Build history of the part. All positions in model axes, mm. A direction names the side the tool comes from. Coordinates: 2 decimals unless noted, no trailing zeros. Write each loop counter-clockwise with the first axis right and the second up, starting at its lowest first coordinate (ties: lowest second). Pieces come first, ordered by that corner, then holes.
from build123d import *
from build123d.topology import SkipClean

# Parameters (mm, degrees)
SKETCH_1_W               = 5
SKETCH_1_H               = 10
EXTRUDE_1_DEPTH          = 5.5
SKETCH_3_W               = 5
SKETCH_3_H               = 46.066203836
SKETCH_3_H_2             = 44
EXTRUDE_2_DEPTH          = 44
CUT_EXTRUDE_1_DEPTH      = 316.357337
CUT_EXTRUDE_1_DEPTH_BACK = 316.357337
SKETCH_4_R               = 8.2
SKETCH_4_R_2             = 1.7
SKETCH_5_R               = 15.5
CUT_EXTRUDE_3_DEPTH      = 1.9
CUT_EXTRUDE_START        = -1.9
SKETCH_6_R               = 15.5
CUT_EXTRUDE_4_DEPTH      = 1.9
CUT_EXTRUDE_5_DEPTH      = 316.357337
CUT_EXTRUDE_5_DEPTH_BACK = 316.357337
SKETCH_7_R               = 8.2
SKETCH_7_R_2             = 1.7
SKETCH_8_R               = 15.5
CUT_EXTRUDE_6_DEPTH      = 1.9
SKETCH_9_R               = 15.5
CUT_EXTRUDE_7_DEPTH      = 1.9
SKETCH_10_W              = 10
SKETCH_10_H              = 34
EXTRUDE_3_DEPTH          = 5
SKETCH_11_W              = 5
SKETCH_11_H              = 41.066203836
SKETCH_11_H_2            = 5
SKETCH_11_H_3            = 44
EXTRUDE_4_DEPTH          = 44
CUT_EXTRUDE_8_DEPTH      = 315.095304008
CUT_EXTRUDE_8_DEPTH_BACK = 315.095304008
SKETCH_12_R              = 1.7
SKETCH_12_R_2            = 8.2
SKETCH_17_W              = 210
SKETCH_17_H              = 49.493882771
EXTRUDE_5_DEPTH          = 7.424621
EXTRUDE_6_DEPTH          = 10
EXTRUDE_8_DEPTH          = 10
SKETCH_20_W              = 40
SKETCH_20_H              = 48.239190952
CUT_EXTRUDE_9_DEPTH      = 10
EXTRUDE_11_DEPTH         = 5
EXTRUDE_13_DEPTH         = 210
FILLET_1_R               = 10
EXTRUDE_14_DEPTH         = 5
SKETCH_26_W              = 25
SKETCH_26_H              = 90
EXTRUDE_15_DEPTH         = 5.5
FILLET_2_R               = 10
CHAMFER_1_SIZE           = 4
CHAMFER_2_SIZE           = 3
FILLET_3_R               = 3


with BuildPart() as part:
    # 草图1 → 凸台-拉伸1 (new body)
    with BuildSketch(Plane(origin=(0, 0, 0), x_dir=(1, 0, 0), z_dir=(0, 1, 0))):
        Polygon((85, -44), (5, -44), (5, -186), (85, -186), (85, -220), (125, -220), (125, -186), (205, -186), (205, -44), (125, -44), (125, -10), (85, -10), align=None)
        Polygon((3, 0), (0, 0), (0, -10), (5, -10), (5, 0), align=None)
        Polygon((5, -10), (0, -10), (0, -220), (5, -220), (5, -186), (5, -44), align=None)
        Polygon((205, 0), (5, 0), (5, -10), (85, -10), (125, -10), (205, -10), align=None)
        Polygon((210, -10), (205, -10), (205, -44), (205, -186), (205, -220), (210, -220), align=None)
        with Locations((207.5, -5)):
            Rectangle(SKETCH_1_W, SKETCH_1_H)
        Polygon((85, -220), (5, -220), (5, -230), (205, -230), (205, -220), (125, -220), align=None)
        with Locations((2.5, -225)):
            Rectangle(SKETCH_1_W, SKETCH_1_H)
        with Locations((207.5, -225)):
            Rectangle(SKETCH_1_W, SKETCH_1_H)
    extrude(amount=EXTRUDE_1_DEPTH)

    # 草图3 → 凸台-拉伸2 (add)
    with BuildSketch(Plane(origin=(0, 5.5, 0), x_dir=(1, 0, 0), z_dir=(0, 1, 0))):
        with Locations((2.5, -28.033101918)):
            Rectangle(SKETCH_3_W, SKETCH_3_H)
        with Locations((2.5, -203)):
            Rectangle(SKETCH_3_W, SKETCH_3_H_2)
        with Locations((207.5, -203)):
            Rectangle(SKETCH_3_W, SKETCH_3_H_2)
        with Locations((207.5, -28.033101918)):
            Rectangle(SKETCH_3_W, SKETCH_3_H)
    extrude(amount=EXTRUDE_2_DEPTH)

    # 草图4 → 切除-拉伸1 (cut, two sides: drawn at the far end of the back side and taken through both)
    with BuildSketch(Plane.ZY.offset(-CUT_EXTRUDE_1_DEPTH_BACK)):
        with Locations((28.033101918, 27.5)):
            Circle(SKETCH_4_R)
        with Locations((28.033101918, 15.6)):
            Circle(SKETCH_4_R_2)
        with Locations((17.727399613, 33.45)):
            Circle(SKETCH_4_R_2)
        with Locations((38.338804223, 33.45)):
            Circle(SKETCH_4_R_2)
    extrude(amount=CUT_EXTRUDE_1_DEPTH + CUT_EXTRUDE_1_DEPTH_BACK, mode=Mode.SUBTRACT)

    # 草图5 → 切除-拉伸3 (cut)
    with BuildSketch(Plane.ZY):
        with Locations((28.033101918, 27.5)):
            Circle(SKETCH_5_R)
    extrude(amount=-CUT_EXTRUDE_3_DEPTH, mode=Mode.SUBTRACT)

    # 草图6 → 切除-拉伸4 (cut)
    with BuildSketch(Plane(origin=(210, 0, 0), x_dir=(0, 0, -1), z_dir=(1, 0, 0)).offset(CUT_EXTRUDE_START)):
        with Locations(Location((-28.033101918, 27.5, 0), (0, 0, 180))):
            Circle(SKETCH_6_R)
    extrude(amount=CUT_EXTRUDE_4_DEPTH, mode=Mode.SUBTRACT)

    # 草图7 → 切除-拉伸5 (cut, two sides: drawn at the far end of the back side and taken through both)
    with BuildSketch(Plane.ZY.offset(-CUT_EXTRUDE_5_DEPTH_BACK)):
        with Locations((203, 27.5)):
            Circle(SKETCH_7_R)
        with Locations((203, 15.6)):
            Circle(SKETCH_7_R_2)
        with Locations((192.694297695, 33.45)):
            Circle(SKETCH_7_R_2)
        with Locations((213.305702305, 33.45)):
            Circle(SKETCH_7_R_2)
    extrude(amount=CUT_EXTRUDE_5_DEPTH + CUT_EXTRUDE_5_DEPTH_BACK, mode=Mode.SUBTRACT)

    # 草图8 → 切除-拉伸6 (cut)
    with BuildSketch(Plane.ZY):
        with Locations((203, 27.5)):
            Circle(SKETCH_8_R)
    extrude(amount=-CUT_EXTRUDE_6_DEPTH, mode=Mode.SUBTRACT)

    # 草图9 → 切除-拉伸7 (cut)
    with BuildSketch(Plane(origin=(210, 0, 0), x_dir=(0, 0, -1), z_dir=(1, 0, 0)).offset(CUT_EXTRUDE_START)):
        with Locations(Location((-203, 27.5, 0), (0, 0, 180))):
            Circle(SKETCH_9_R)
    extrude(amount=CUT_EXTRUDE_7_DEPTH, mode=Mode.SUBTRACT)

    # 草图10 → 凸台-拉伸3 (add)
    with BuildSketch(Plane(origin=(0, 5.5, 0), x_dir=(1, 0, 0), z_dir=(0, 1, 0))):
        with Locations((200, -27)):
            Rectangle(SKETCH_10_W, SKETCH_10_H)
        with Locations((10, -27)):
            Rectangle(SKETCH_10_W, SKETCH_10_H)
        with Locations((10, -203)):
            Rectangle(SKETCH_10_W, SKETCH_10_H)
        with Locations((200, -203)):
            Rectangle(SKETCH_10_W, SKETCH_10_H)
    extrude(amount=-EXTRUDE_3_DEPTH)

    # 草图11 → 凸台-拉伸4 (add)
    with BuildSketch(Plane(origin=(0, 5.5, 0), x_dir=(1, 0, 0), z_dir=(0, 1, 0))):
        with Locations((7.5, -30.533101918)):
            Rectangle(SKETCH_11_W, SKETCH_11_H)
        with Locations((7.5, -7.5)):
            Rectangle(SKETCH_11_W, SKETCH_11_H_2)
        with Locations((202.5, -7.5)):
            Rectangle(SKETCH_11_W, SKETCH_11_H_2)
        with Locations((202.5, -30.533101918)):
            Rectangle(SKETCH_11_W, SKETCH_11_H)
        with Locations((7.5, -203)):
            Rectangle(SKETCH_11_W, SKETCH_11_H_3)
        with Locations((202.5, -203)):
            Rectangle(SKETCH_11_W, SKETCH_11_H_3)
    extrude(amount=EXTRUDE_4_DEPTH)

    # 草图12 → 切除-拉伸8 (cut, two sides: drawn at the far end of the back side and taken through both)
    with BuildSketch(Plane.ZY.offset(-1.9).offset(-CUT_EXTRUDE_8_DEPTH_BACK)):
        with Locations(Location((17.727399613, 33.45, 0), (0, 0, 180))):
            Circle(SKETCH_12_R)
        with Locations(Location((38.338804223, 33.45, 0), (0, 0, 180))):
            Circle(SKETCH_12_R)
        with Locations(Location((28.033101918, 15.6, 0), (0, 0, 180))):
            Circle(SKETCH_12_R)
        with Locations(Location((28.033101918, 27.5, 0), (0, 0, 180))):
            Circle(SKETCH_12_R_2)
        with Locations(Location((192.694297695, 33.45, 0), (0, 0, 180))):
            Circle(SKETCH_12_R)
        with Locations(Location((213.305702305, 33.45, 0), (0, 0, 180))):
            Circle(SKETCH_12_R)
        with Locations(Location((203, 15.6, 0), (0, 0, 180))):
            Circle(SKETCH_12_R)
        with Locations(Location((203, 27.5, 0), (0, 0, 180))):
            Circle(SKETCH_12_R_2)
    extrude(amount=CUT_EXTRUDE_8_DEPTH + CUT_EXTRUDE_8_DEPTH_BACK, mode=Mode.SUBTRACT)

    # 草图17 → 凸台-拉伸5 (add, through all)
    with BuildSketch(Plane(origin=(0, 5.25, 5.25), x_dir=(1, 0, 0), z_dir=(0, 0.7071067811865464, 0.7071067811865487))):
        with Locations((105, 25.100494776)):
            Rectangle(SKETCH_17_W, SKETCH_17_H)
    extrude(amount=-EXTRUDE_5_DEPTH)

    # 草图18 → 凸台-拉伸6 (add)
    with BuildSketch(Plane.ZY):
        Polygon((-29.997460135, 40.497460135), (5, 40.5), (5, 5.5), align=None)
    extrude(amount=-EXTRUDE_6_DEPTH)

    # 草图19 → 凸台-拉伸8 (add)
    with BuildSketch(Plane(origin=(210, 0, 0), x_dir=(0, 0, -1), z_dir=(1, 0, 0))):
        Polygon((30, 40.5), (-5, 40.5), (-5, 5.5), align=None)
    extrude(amount=-EXTRUDE_8_DEPTH)

    # 草图20 → 切除-拉伸9 (cut)
    with BuildSketch(Plane(origin=(0, 5.25, 5.25), x_dir=(1, 0, 0), z_dir=(0, 0.7071067811865465, 0.7071067811865487))):
        Polygon((85, 49.847436162), (15, 49.847436162), (85, 1.60824521), align=None)
        with Locations((105, 25.727840686)):
            Rectangle(SKETCH_20_W, SKETCH_20_H)
        Polygon((125, 49.847436162), (125, 1.60824521), (195, 49.847436162), align=None)
    extrude(amount=-CUT_EXTRUDE_9_DEPTH, mode=Mode.SUBTRACT)

    # 草图21 → 凸台-拉伸11 (add)
    with BuildSketch(Plane(origin=(0, 5.5, 0), x_dir=(1, 0, 0), z_dir=(0, 1, 0))):
        Polygon((15, -44), (32.5, -10), (15, -10), align=None)
        Polygon((67.5, -10), (32.5, -10), (41.25, -27), (50, -44), (58.75, -27), align=None)
        Polygon((50, -44), (41.25, -27), (41.25, -44), align=None)
        Polygon((58.75, -27), (50, -44), (58.75, -44), align=None)
        Polygon((85, -10), (67.5, -10), (85, -44), align=None)
        Polygon((125, -10), (125, -44), (142.5, -10), align=None)
        Polygon((177.5, -10), (142.5, -10), (151.25, -27), (160, -44), (168.75, -27), align=None)
        Polygon((195, -10), (177.5, -10), (195, -44), align=None)
        Polygon((168.75, -27), (160, -44), (168.75, -44), align=None)
        Polygon((151.25, -27), (151.25, -44), (160, -44), align=None)
    extrude(amount=-EXTRUDE_11_DEPTH)

    # 草图22 → 凸台-拉伸13 (add)
    with SkipClean():  # the faces are left unmerged after this step: merging them gives an invalid solid
        with BuildSketch(Plane.ZY):
            Polygon((0, 0.5), (0, 0), (-0.25, 0.25), align=None)
        extrude(amount=-EXTRUDE_13_DEPTH)

    # 圆角1
    # the kernel refuses this fillet: 10 mm, written as the material it takes off along each edge
    with BuildSketch(Plane(origin=(220.355339059, 0, 0), x_dir=(0, 0, 1), z_dir=(-1, 0, 0))) as fillet_1_piece_1:
        with BuildLine():
            CenterArc((FILLET_1_R * 0.414213562373, FILLET_1_R), FILLET_1_R, 225, 45)
            Line((-FILLET_1_R * 0.292893218813, FILLET_1_R * 0.292893218813), (0, 0))
            Line((0, 0), (FILLET_1_R * 0.414213562373, 0))
        make_face()
    extrude(amount=230.710678119, mode=Mode.SUBTRACT)

    # 草图23 → 凸台-拉伸14 (add)
    with BuildSketch(Plane(origin=(0, 5.5, 0), x_dir=(1, 0, 0), z_dir=(0, 1, 0))):
        Polygon((23.75, -27), (23.75, -44), (15, -44), align=None)
        Polygon((76.25, -27), (76.25, -44), (85, -44), align=None)
        Polygon((133.75, -27), (133.75, -44), (125, -44), align=None)
        Polygon((186.25, -27), (186.25, -44), (195, -44), align=None)
    extrude(amount=-EXTRUDE_14_DEPTH)

    # 草图26 → 凸台-拉伸15 (add)
    with BuildSketch(Plane(origin=(0, 5.5, 0), x_dir=(1, 0, 0), z_dir=(0, 1, 0))):
        with Locations((-12.5, -116.033101918)):
            Rectangle(SKETCH_26_W, SKETCH_26_H)
        with Locations((222.5, -116.033101918)):
            Rectangle(SKETCH_26_W, SKETCH_26_H)
    extrude(amount=-EXTRUDE_15_DEPTH)

    # 圆角2
    fillet_2_edges = [part.edges().sort_by_distance(p)[0] for p in [
        (0, 2.75, 161.033101918),
        (-25, 2.75, 161.033101918),
        (-25, 2.75, 71.033101918),
        (0, 2.75, 71.033101918),
        (235, 2.75, 161.033101918),
        (210, 2.75, 161.033101918),
        (210, 2.75, 71.033101918),
        (235, 2.75, 71.033101918),
    ]]
    fillet(fillet_2_edges, radius=FILLET_2_R)

    # 倒角1
    chamfer_1_edges = [part.edges().sort_by_distance(p)[0] for p in [
        (15, 3, 186),
        (15, 3, 220),
        (195, 3, 220),
        (195, 3, 186),
        (85, 2.75, 220),
        (85, 2.75, 186),
        (125, 2.75, 186),
        (125, 2.75, 220),
    ]]
    chamfer(chamfer_1_edges, length=CHAMFER_1_SIZE)

    # 倒角2
    chamfer_2_edges = [part.edges().sort_by_distance(p)[0] for p in [
        (58.75, 3, 44),
        (41.25, 3, 44),
        (168.75, 3, 44),
        (151.25, 3, 44),
        (23.75, 3, 44),
        (76.25, 3, 44),
        (133.75, 3, 44),
        (186.25, 3, 44),
    ]]
    chamfer(chamfer_2_edges, length=CHAMFER_2_SIZE)

    # 圆角3
    fillet_3_edges = [part.edges().sort_by_distance(p)[0] for p in [
        (32.5, 3, 10),
        (67.5, 3, 10),
        (142.5, 3, 10),
        (177.5, 3, 10),
    ]]
    fillet(fillet_3_edges, radius=FILLET_3_R)


solid = part.part
(1) Flat gauge pins, fed straight in: P1, Ø1.5, axis at x = -12, y = 4, coming from the -Z side; P2, Ø7, axis at x = 3.5, y = 43, coming from the -Z side; P3, Ø12, axis at y = 8.5, z = 177, coming from the +X side. Where does each tip first touch, or does it go through?
(2) Slice it at B-B, the plane z = 143. List the corners of the cut face in (x, y), and give its area (3 significant figures).
(3) Slice it at A-A, the plane x = 55. List the corners of the cut face in (y, z), and give its area (3 significant figures).
(4) Probe L1, parallel to Z at x = 8.45, y = 15.6; L2, parallel to Z at x = 1, y = 27; L3, parallel to Y at x = 1, z = 202. List the from-to ranges inside material, lowest first.
(5) 3-axis set-ups, long thin cutter, end or side, ignore diameter. For faces 1 (the flat face through (200, 33, 20)), 2 (the flat face through (26.75, 3.04, 21.17)), 3 (the flat face through (208.1, 34, 210)), 4 (the flat face through (5, 27, 51.066)): which of +Z, -Z, +X, -X, +Y, -Y reach the whole face in a straight line?
(6) Two-plate mould, pull along X, no slides. Class faces 5 (the flat face through (5, 27, 225)), 6 (the cylindrical face through (213.01, 2.71, 163.88)), 7 (the cylindrical face through (-21.993, 2.712, 158.181)), 8 (the flat face through (10, 0.5, 203)): pulls with the +X half, pulls with the -X half, needs draft (parallel to the pull), parting line crosses it, or undercut.
(7) Slice it at C-C, the plane x = -7. List the corners of the cut face in (y, z), and give its area (3 significant figures).
Results:
1. P1: stops at z = 71.03
1. P2: stops at z = -30.99
1. P3: stops at x = 210
2. outline: (-25, 0) - (235, 0) - (235, 5.5) - (-25, 5.5) - close
2. area: 1,430 mm2
3. outline: (0, 4.14) arc R10 ccw to (2.93, -2.93) - (15.76, -15.76) - (21.01, -10.51) - (5.5, 5) - (5.5, 186) - (0, 186) - (0, 44) - (0.5, 44) - (0.5, 10) - (0, 10) - close; (0, 220) - (5.5, 220) - (5.5, 230) - (0, 230) - close
3. area: 1,210 mm2
4. L1: z = -15.6 to 26.33, 29.73 to 51.07, 181 to 201.3, 204.7 to 225
4. L2: z = -27 to 12.54, 43.53 to 51.07, 181 to 187.51, 218.49 to 225
4. L3: y = 0 to 12.03, 42.97 to 49.5
5. face 1: +Z, +Y
5. face 2: +Y, -Y
5. face 3: +X
5. face 4: +X, -X, +Y
6. face 5: needs draft
6. face 6: pulls with the +X half
6. face 7: pulls with the -X half
6. face 8: undercut
7. outline: (0, 70.57) - (5.5, 70.57) - (5.5, 161.49) - (0, 161.49) - close
7. area: 500 mm2
